Geometry check sheet. Reference: the model listing, model coordinates, mm. Face numbers are marked on the shaded views. Give positions to 0.01 mm unless a question says otherwise; leave off trailing zeros. Order: outer loops, then holes, each group sorted by start corner. A loop starts at its lowest first (then second) coordinate and runs counter-clockwise, first axis right, second up.
from build123d import *

# Parameters (mm, degrees)
SKETCH1_R           = 19
SKETCH1_R_2         = 17
BOSS_EXTRUDE1_DEPTH = 240
SKETCH2_R           = 20
SKETCH2_R_2         = 19
BOSS_EXTRUDE2_DEPTH = 30


with BuildPart() as part:
    # Sketch1 → Boss-Extrude1 (new body)
    with BuildSketch(Plane(origin=(0, 0, 0), x_dir=(0, 0, -1), z_dir=(1, 0, 0))):
        Circle(SKETCH1_R)
        Circle(SKETCH1_R_2, mode=Mode.SUBTRACT)
    extrude(amount=BOSS_EXTRUDE1_DEPTH)

    # Sketch2 → Boss-Extrude2 (add, symmetric)
    with BuildSketch(Plane(origin=(240, 0, 0), x_dir=(0, 0, -1), z_dir=(1, 0, 0))):
        Circle(SKETCH2_R)
        Circle(SKETCH2_R_2, mode=Mode.SUBTRACT)
    extrude(amount=BOSS_EXTRUDE2_DEPTH, both=True)


solid = part.part
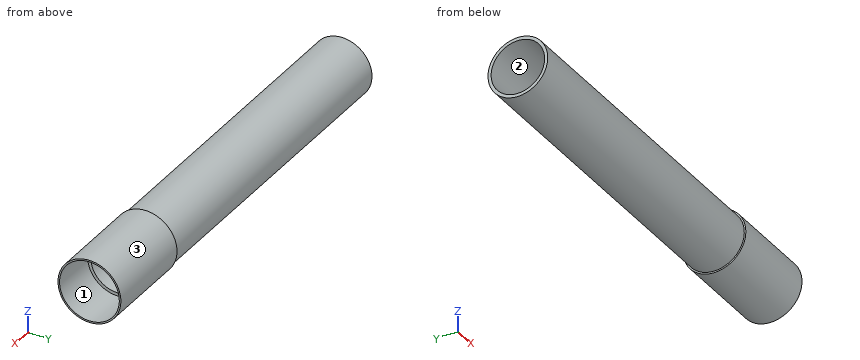
Item 1: Sectioned sample at D-D (x = 221.5). Enter the section's corners in (y, z).
Reported:
outline: circle Ø40 at (0, 0); hole circle Ø34 at (0, 0)
Item 2: Gauge pin test, flat ends, axial feed: pin 1 (12 mm diameter, centred on x = 61.5, y = 12.5, fed in from -Z); pin 2 (2 mm diameter, centred on x = 137.5, y = 14, fed in from +Z); pin 3 (6 mm diameter, centred on y = -13.5, z = -7.5, fed in from -X); pin 4 (2 mm diameter, centred on x = 216, y = 10, fed in from +Z). Record the tip position at first contact, or that the pin passes through.
Reported:
pin 1: stops at z = -17.85
pin 2: stops at z = 13.86
pin 3: stops at x = 0
pin 4: stops at z = 17.86
Item 3: Sectioned sample at C-C (x = 96). Enter the section's corners in (y, z), and give its area (3 significant figures).
Reported:
outline: circle Ø38 at (0, 0); hole circle Ø34 at (0, 0)
area: 226 mm2
Item 4: Sectioned sample at A-A (y = 0). Enter the section's corners in (x, z), and give its area (3 significant figures).
Reported:
outline: (0, -19) - (210, -19) - (210, -20) - (270, -20) - (270, -19) - (240, -19) - (240, -17) - (0, -17) - close; (0, 17) - (240, 17) - (240, 19) - (270, 19) - (270, 20) - (210, 20) - (210, 19) - (0, 19) - close
area: 1,080 mm2
Item 5: Scan lines: L1, parallel to Y at x = 17, z = 0.5; L2, parallel to Y at x = 32.5, z = -8.5; L3, parallel to Z at x = 218, y = -13. Record each from-to range of solid material in increasing order.
Reported:
L1: y = -18.99 to -16.99, 16.99 to 18.99
L2: y = -16.99 to -14.72, 14.72 to 16.99
L3: z = -15.2 to -10.95, 10.95 to 15.2
Item 6: Draft check along Y on the marked faces 1, 2 and 3. Enter one of: released by +Y, released by -Y, zero draft, split by the parting line, or undercut.
Reported:
face 1: undercut
face 2: undercut
face 3: split by the parting line
